Here's how the part is built. I have some questions about the finished solid (model axes, mm). Face numbers are marked on the shaded views. A direction names the side the tool comes from. Coordinates: 2 decimals unless noted, no trailing zeros. Loops run counter-clockwise (first coordinate to the right, second up) from the corner with the lowest first, then second, coordinate; pieces in that order, holes last. Notation, with made-up numbers: M 55,-24.5 L 103,-24.5 A26 cw 103,7.5 Z; hole C 68.25,44 d3. An arc over 180 degrees is marked long. Use one line per item in the form item = value. Start each with the question number.
(1) Will these pins go through, and if not, where does the flat tip stop? P1, Ø8, axis at y = 8, z = 2.5, coming from the +X side; P2, Ø5, axis at x = 7.5, z = -3.5, coming from the +Y side.
(2) Imagine slicing it at D-D, the plane y = 5.5. Please give me the cut outline in (x, z), and give its area (3 significant figures).
(3) Imagine slicing it at A-A, the plane x = 10. Please give me the cut outline in (y, z), and give its area (3 significant figures).
(4) On a 3-axis mill with a long thin cutter (end or side, diameter ignored), from which of +Z, -Z, +X, -X, +Y, -Y can I reach the whole of each face in a straight line? I mean the marked faces 1 and 2. Say none if no direction works.
(5) Imagine slicing it at C-C, the plane z = 0.5. Please give me the cut outline in (x, y).
(6) Please list where these lines run through material, in increasing order: L1, parallel to X at y = 1.1, z = 0; L2, parallel to Z at x = 7, y = 8.25.
```python
from build123d import *

# Parameters (mm, degrees)
BOSS_EXTRUDE1_DEPTH = 10
SKETCH2_W           = 18
SKETCH2_H           = 16
CUT_EXTRUDE1_DEPTH  = 18
SKETCH3_R           = 3
CUT_EXTRUDE2_DEPTH  = 20
SKETCH4_R           = 3
CUT_EXTRUDE3_DEPTH  = 20


with BuildPart() as part:
    # Sketch1 → Boss-Extrude1 (new, symmetric)
    with BuildSketch(Plane.XY):
        Polygon((20, 0), (0, 0), (0, 20), (2, 20), (20, 2), align=None)
    extrude(amount=BOSS_EXTRUDE1_DEPTH, both=True)

    # Sketch2 → Cut-Extrude1 (cut)
    with BuildSketch(Plane(origin=(0, 20, 0), x_dir=(1, 0, 0), z_dir=(0, 1, 0))):
        with Locations((11, 0)):
            Rectangle(SKETCH2_W, SKETCH2_H)
    extrude(amount=-CUT_EXTRUDE1_DEPTH, mode=Mode.SUBTRACT)

    # Sketch3 → Cut-Extrude2 (cut)
    with BuildSketch(Plane(origin=(2, 0, 0), x_dir=(0, 0, -1), z_dir=(1, 0, 0))):
        with Locations((0, 10)):
            Circle(SKETCH3_R)
    extrude(amount=-CUT_EXTRUDE2_DEPTH, mode=Mode.SUBTRACT)

    # Sketch4 → Cut-Extrude3 (cut)
    with BuildSketch(Plane(origin=(0, 2, 0), x_dir=(1, 0, 0), z_dir=(0, 1, 0))):
        with Locations(Location((10, 0, 0), (0, 0, 270))):
            Circle(SKETCH4_R)
    extrude(amount=-CUT_EXTRUDE3_DEPTH, mode=Mode.SUBTRACT)


solid = part.part
```
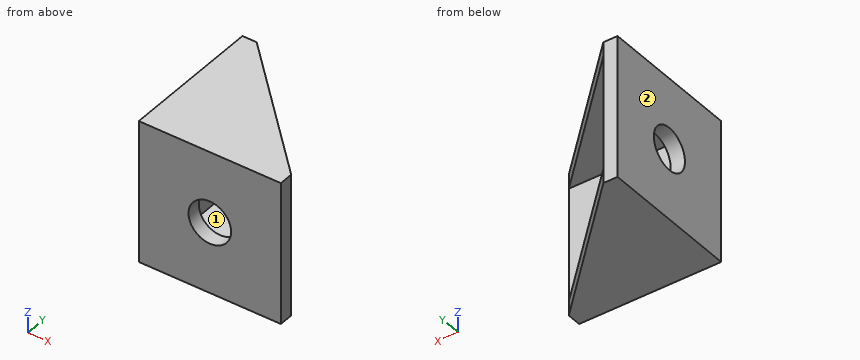
Answer:
q1.P1 = 2
q1.P2 = 2
q2.outline = M 0,-10 L 16.5,-10 L 16.5,-8 L 2,-8 L 2,8 L 16.5,8 L 16.5,10 L 0,10 Z
q2.area = 98.0 mm²
q3.outline = M 0,-10 L 12,-10 L 12,-8 L 2,-8 L 2,-3 L 0,-3 Z; M 0,3 L 2,3 L 2,8 L 12,8 L 12,10 L 0,10 Z
q3.area = 68.0 mm²
q4.face_1 = +X, +Y
q4.face_2 = +Z, -Z, -X, +Y, -Y
q5.outline = M 0,0 L 7.04,0 L 7.04,2 L 2,2 L 2,7.04 L 0,7.04 Z; M 0,12.96 L 2,12.96 L 2,20 L 0,20 Z; M 12.96,0 L 20,0 L 20,2 L 12.96,2 Z
q6.L1 = 0 to 7, 13 to 20
q6.L2 = -10 to -8, 8 to 10
